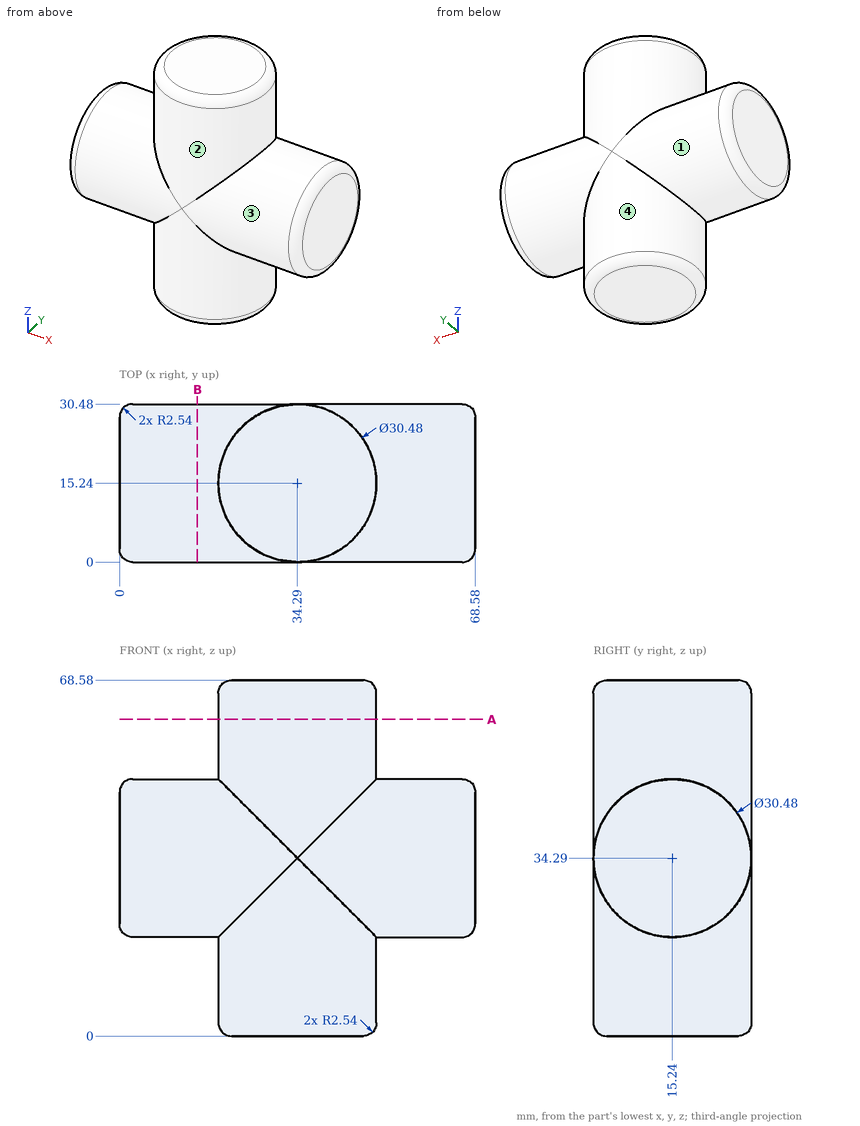
Study the drawing (mm; zero at the part's minimum x, y, z) and answer. A direction names the side the tool comes from. Give positions to 0.01 mm unless a question says otherwise; leave off trailing zeros. Write each loop counter-clockwise with the first axis right and the second up, starting at its lowest first coordinate (ties: lowest second). Pieces come first, ordered by that corner, then holes. Notation, with made-up numbers: (-27.5, 31.25) - (0.5, 31.25) arc R32 cw to (0.5, 62.25) - close; hole circle Ø5 at (17, -23.5). An arc over 180 degrees is marked (long way). One line per question, with ' | ' between items. Start each with the question number.
1. For the marked faces 1, 2, 3 and 4, determine the directions among +Z, -Z, +X, -X, +Y, -Y from which every point of the face is accessible in a straight line to the end or side of a thin tool.
2. Section B-B, the plane x = 15 is taken. Determine the outline of the cut face in (y, z).
3. Section A-A, the plane z = 61 is taken. Determine the outline of the cut face in (x, y), then the cut area to 3 significant figures.
4. Given P1, Ø10, axis at y = 24, z = 59, coming from the -X side; P2, Ø1.5, axis at x = 44, z = 53.5, coming from the -Y side; P3, Ø5, axis at x = 16, y = 7.5, coming from the +Z side, each flat-ended and moving along its own axis, determine where each tip first touches the part or whether it passes through.
5. Straight lines are drawn through the part: line 1 (Z direction, x = 9.5, y = 16); line 2 (Z direction, x = 46.5, y = 11); line 3 (Y direction, x = 48, z = 34). For each, find the intervals that lie inside material, in ascending order.
Result:
1) face 1: -X | face 2: +Z | face 3: +X | face 4: -Z
2) outline: circle Ø30.48 at (15.24, 34.29)
3) outline: circle Ø30.48 at (34.29, 15.24) | area: 730 mm2
4) P1: stops at x = 19.52 | P2: stops at y = 2.91 | P3: stops at z = 48.6
5) line 1: z = 19.07 to 49.51 | line 2: z = 0.01 to 68.57 | line 3: y = 0 to 30.48
